Read the model definition and answer for the solid it produces. Units are mm, in the model's axes. A direction names the side the tool comes from. Round coordinates to 2 decimals unless told otherwise and drop trailing zeros. Order: outer loops, then holes, each group sorted by start corner. A loop starts at its lowest first (then second) coordinate and runs counter-clockwise, first axis right, second up.
from build123d import *

# Parameters (mm, degrees)
SKETCH1_R           = 3.429
BOSS_EXTRUDE1_DEPTH = 3.175
SKETCH2_W           = 12.7
SKETCH2_H           = 12.446
BOSS_EXTRUDE2_DEPTH = 9.525


with BuildPart() as part:
    # Sketch1 → Boss-Extrude1 (new body, symmetric)
    with BuildSketch(Plane.XY):
        with BuildLine():
            Line((0, 12.7), (38.1, 12.7))
            Line((38.1, 12.7), (38.1, 0.254))
            Line((38.1, 0.254), (12.697459746, 0.254))
            ThreePointArc((12.697459746, 0.254), (-8.89, -9.069614104), (0, 12.7))
        make_face()
        Circle(SKETCH1_R, mode=Mode.SUBTRACT)
    extrude(amount=BOSS_EXTRUDE1_DEPTH, both=True)

    # Sketch2 → Boss-Extrude2 (add, symmetric)
    with BuildSketch(Plane.XY):
        with Locations((31.75, 6.477)):
            Rectangle(SKETCH2_W, SKETCH2_H)
    extrude(amount=BOSS_EXTRUDE2_DEPTH, both=True)


solid = part.part
Q1. A cutting plane is placed at D-D, the plane z = 6.5. Give the vertices of the cut face in (x, y), plus the area to 3 significant figures.
Outcome:
outline: (25.4, 0.25) - (38.1, 0.25) - (38.1, 12.7) - (25.4, 12.7) - close
area: 158 mm2
Q2. Straight lines are drawn through the part: probe 1 along Y at (x, z) = (0, -2); probe 2 along X at (y, z) = (5.5, 3.25); probe 3 along Y at (x, z) = (20, -0.5). For each, find the intervals that lie inside material, in ascending order.
Outcome:
probe 1: y = -12.7 to -3.43, 3.43 to 12.7
probe 2: x = 25.4 to 38.1
probe 3: y = 0.25 to 12.7
Q3. A cutting plane is placed at C-C, the plane y = -2.5. Give the vertices of the cut face in (x, z) (1 decimal).
Outcome:
outline: (-12.5, -3.2) - (-2.3, -3.2) - (-2.3, 3.2) - (-12.5, 3.2) - close; (2.3, -3.2) - (12.5, -3.2) - (12.5, 3.2) - (2.3, 3.2) - close
Q4. A cutting plane is placed at A-A, the plane x = 1. Give the vertices of the cut face in (y, z) (3 decimals).
Outcome:
outline: (-12.661, -3.175) - (-3.28, -3.175) - (-3.28, 3.175) - (-12.661, 3.175) - close; (3.28, -3.175) - (12.7, -3.175) - (12.7, 3.175) - (3.28, 3.175) - close
Q5. A cutting plane is placed at B-B, the plane z = -1.5. Give the vertices of the cut face in (x, y), plus the area to 3 significant figures.
Outcome:
outline: (0, 12.7) arc R12.7 ccw (long way) to (12.7, 0.25) - (38.1, 0.25) - (38.1, 12.7) - close; hole circle Ø6.86 at (0, 0)
area: 821 mm2
Q6. For faces 4 (the face through (23, 12.7, 0)), 5 (the face through (25.4, 6, -6)), 6 (the face through (7, 3, 3.175)), determine the directions among +Z, -Z, +X, -X, +Y, -Y from which every point of the face is accessible in a straight line to the end or side of a thin tool.
Outcome:
face 4: +Z, -Z, +X, -X, +Y
face 5: -Z, -X, +Y, -Y
face 6: +Z, -X, +Y, -Y
Q7. Flat-ended cylindrical pins translate along their axes: pin 1 (10 mm diameter, centred on x = 3, y = -7, fed in from +Z) (3 decimals); pin 2 (2 mm diameter, centred on x = 24, z = -3, fed in from -Y); pin 3 (1 mm diameter, centred on x = -0.5, y = 8.5, fed in from -Z) (3 decimals). Find the tip coordinate at first contact, or state that the pin passes through.
Outcome:
pin 1: stops at z = 3.175
pin 2: stops at y = 0.25
pin 3: stops at z = -3.175
Q8. For a pull along Y with two mould halves and no side action, classify faces 1 (the face through (-0.74, -3.35, -0.04)), 2 (the face through (28, 0.254, 0)), 3 (the face through (38.1, 6, 0)) as released by +Y, released by -Y, zero draft, split by the parting line, or undercut.
Outcome:
face 1: undercut
face 2: released by -Y
face 3: zero draft
